Autodesk Inventor part; units mm, degrees
ref_plane "Arbeitsebene1" through (0, 0, 48) normal (0, 0, 1) x (1, 0, 0)
ref_plane "YZ Plane" through (0, 0, 0) normal (1, 0, 0) x (0, 1, 0)
ref_plane "XZ Plane" through (0, 0, 0) normal (0, 1, 0) x (-1, 0, 0)
sketch "Skizze1" plane through (0, 0, 0) normal (0, 0, 1) x (1, 0, 0)
  line L0 (0, 45) -> (110, 45)
  line L1 (110, 45) -> (110, 0)
  line L2 (110, 0) -> (0, 0)
  line L3 (0, 0) -> (0, 45)
  dimension "d0" = 110
  dimension "d1" = 45
extrude "Extrusion1" add sketch "Skizze1" along normal blind 12
sketch "Skizze2" plane through (110, 0, 0) normal (1, 0, 0) x (0, 0, -1)
  line L0 (0, 45) -> (-12, 45)
  line L1 (0, 45) -> (-62, 45)
  line L2 (-62, 45) -> (-62, 33)
  line L3 (-62, 33) -> (0, 33)
  line L4 (0, 33) -> (0, 45)
  point P0 (0, 0)
  dimension "d4" = 12
  dimension "d5" = 62
extrude "Extrusion2" add sketch "Skizze2" against normal up to surface (110 mm away)
fillet "Rundung1" radius 12 4 edges at (110, 0, 6) (0, 0, 6) (0, 39, 62) (110, 39, 62)
ref_plane "Arbeitsebene1" through (0, 0, 48) normal (0, 0, 1) x (1, 0, 0)
sketch "Skizze5" plane through (0, 0, 48) normal (0, 0, 1) x (1, 0, 0)
  line L0 (110, 45) -> (0, 45)
  line L1 (30, 45) -> (80, 45)
  line L2 (80, 45) -> (80, 10)
  line L3 (80, 10) -> (30, 10)
  line L4 (30, 10) -> (30, 45)
  line L5 (12, 0) -> (98, 0)
  point P0 (0, 0)
  point P1 (55, 10)
  point P2 (55, 0)
  dimension "d12" = 50
  dimension "d13" = 35
extrude "Extrusion4" add sketch "Skizze5" along normal up to surface (14 mm away)
sketch "Skizze3" plane through (0, 0, 12) normal (0, 0, 1) x (1, 0, 0)
  line L0 (98, 33) -> (12, 33)
  line L1 (44, 33) -> (66, 33)
  line L2 (66, 33) -> (66, 10)
  line L3 (66, 10) -> (44, 10)
  line L4 (44, 10) -> (44, 33)
  line L5 (12, 0) -> (98, 0)
  point P0 (0, 0)
  point P1 (55, 10)
  point P2 (55, 0)
  dimension "d9" = 22
  dimension "d10" = 23
sketch "Skizze9" plane through (0, 0, 48) normal (0, 0, -1) x (-1, 0, 0)
  line L0 (-80, 10) -> (-30, 10)
  line L1 (-35, 33) -> (-75, 33)
  line L2 (-75, 33) -> (-75, 10)
  line L3 (-75, 10) -> (-35, 10)
  line L4 (-35, 10) -> (-35, 33)
  line L5 (-98, 45) -> (-12, 45)
  point P0 (0, 0)
  point P1 (-55, 33)
  point P2 (-55, 45)
  dimension "d30" = 40
  dimension "d31" = 23
loft "Erhebung3" add profiles "Skizze3", "Skizze9"
sketch "Skizze10" plane through (30, 10, 62) normal (0, -1, 0) x (1, 0, 0)
  line L0 (68, 0) -> (-18, 0)
  arc A0 (10, 0) -> (40, 0) centre (25, 0) ccw
  line L1 (0, -14) -> (0, 0)
  line L2 (50, -14) -> (50, 0)
  point P0 (-30, -62)
  dimension "d38" = 30
  dimension "d39" = 10
extrude "Extrusion5" cut sketch "Skizze10" against normal up to surface (35 mm away)
sketch "Skizze11" plane through (0, 33, 12) normal (0, -1, 0) x (1, 0, 0)
  arc A0 (12, 50) -> (0, 38) centre (12, 38) ccw
  point P0 (0, -12)
hole "Bohrung1" at (12, 33, 50) direction (0, 1, 0) diameter 12 depth 12
sketch "Skizze12" plane through (110, 33, 12) normal (0, -1, 0) x (1, 0, 0)
  arc A0 (0, 38) -> (-12, 50) centre (-12, 38) ccw
  point P0 (-110, -12)
hole "Bohrung2" at (98, 33, 50) direction (0, 1, 0) diameter 12 depth 12
sketch "Skizze13" plane through (0, 0, 12) normal (0, 0, 1) x (1, 0, 0)
  arc A0 (98, 0) -> (110, 12) centre (98, 12) ccw
  point P0 (0, 0)
hole "Bohrung3" at (98, 12, 12) direction (0, 0, -1) diameter 12 depth 12
sketch "Skizze14" plane through (0, 0, 12) normal (0, 0, 1) x (1, 0, 0)
  arc A0 (0, 12) -> (12, 0) centre (12, 12) ccw
  point P0 (0, 0)
hole "Bohrung4" at (12, 12, 12) direction (0, 0, -1) diameter 12 depth 12
sketch "Skizze15" plane through (12, 0, 0) normal (0, -1, 0) x (1, 0, 0)
  line L0 (0, 0) -> (86, 0)
  line L1 (13, 0) -> (73, 0)
  line L2 (73, 0) -> (73, 8)
  line L3 (73, 8) -> (13, 8)
  line L4 (13, 8) -> (13, 0)
  line L5 (-12, 12) -> (-12, 0)
  dimension "d70" = 60
  dimension "d71" = 25
  dimension "d72" = 8
extrude "Extrusion6" cut sketch "Skizze15" against normal up to surface (45 mm away)
properties part number "manu" material "Stahl, galvanisiert"
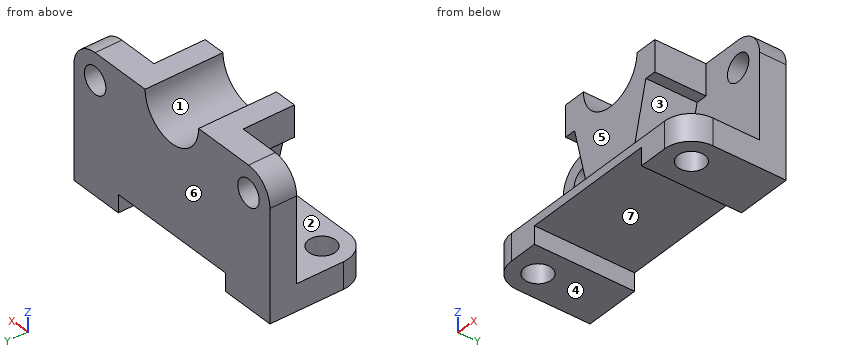
CAD build for the part. Positions are in the model's coordinates, mm. Face numbers are marked on the shaded views. A direction names the side the tool comes from. Coordinates: 2 decimals unless noted, no trailing zeros. Write each loop counter-clockwise with the first axis right and the second up, starting at its lowest first coordinate (ties: lowest second). Pieces come first, ordered by that corner, then holes. Notation, with made-up numbers: (-6, 83.5) -> (-1, 83.5) arc R23 cw to (-1, 122.5) -> close; hole circle Ø3 at (53, -10.75). An arc over 180 degrees is marked (long way). Return JSON: item names as keys, results as strings. Group by question number.
Q1. Cut at B-B, the plane y = 31. Give the cut face in (x, z).
Q2. Cut at C-C, the plane z = 31. Give the cut face in (x, y).
Q3. Pull direction Z, two halves, no side cores. Call the marked faces 1, 2, 3 and 4: released by +Z, released by -Z, zero draft, split by the parting line, or undercut.
Q4. Which spindle directions (+Z, -Z, +X, -X, +Y, -Y) get a long thin tool onto all of the face, cutting with end or side? Do the marked faces 5, 6 and 7. Say none if no direction does.
Q5. Drill centre lines: line 1 (X direction, y = 12, z = 9); line 2 (Y direction, x = 98, z = 6); line 3 (X direction, y = 42, z = 50). Where is each one in solid material? Low to high.
Q6. Cut at D-D, the plane x = 16. Give the cut face in (y, z), then the cut area to 3 significant figures.
Q7. Cut at A-A, the plane z = 6.5. Give the cut face in (x, y).
Q8. Flat gauge pins, fed straight in: pin 1 (1.5 mm diameter, centred on x = 33.5, y = 23.5, fed in from -Z); pin 2 (7 mm diameter, centred on x = 12, y = 12, fed in from +Z); pin 3 (19 mm diameter, centred on x = 98, y = 12, fed in from +Z); pin 4 (10 mm diameter, centred on x = 72, z = 53, fed in from -Y). Where does each tip first touch, or does it go through?
Returned:
{
 "1": {"outline": "(0, 0) -> (25, 0) -> (25, 8) -> (85, 8) -> (85, 0) -> (110, 0) -> (110, 12) -> (66, 12) -> (75, 48) -> (80, 48) -> (80, 62) -> (70, 62) arc R15 cw to (40, 62) -> (30, 62) -> (30, 48) -> (35, 48) -> (44, 12) -> (0, 12) -> close"},
 "2": {"outline": "(0, 33) -> (39.25, 33) -> (39.25, 10) -> (70.75, 10) -> (70.75, 33) -> (110, 33) -> (110, 45) -> (0, 45) -> close"},
 "3": {"face 1": "released by +Z", "face 2": "undercut", "face 3": "undercut", "face 4": "released by -Z"},
 "4": {"face 5": "+Z, +X, -X, -Y", "face 6": "+Z, -Z, +X, -X, +Y", "face 7": "-Z, +Y, -Y"},
 "5": {"line 1": "x = 0 to 6, 18 to 92, 104 to 110", "line 2": "y = 0 to 6, 18 to 45", "line 3": "x = 0 to 6, 18 to 46, 64 to 92, 104 to 110"},
 "6": {"outline": "(0, 0) -> (7.53, 0) -> (7.53, 12) -> (0, 12) -> close; (16.47, 0) -> (45, 0) -> (45, 45.53) -> (33, 45.53) -> (33, 12) -> (16.47, 12) -> close; (33, 54.47) -> (45, 54.47) -> (45, 62) -> (33, 62) -> close", "area": "925 mm2"},
 "7": {"outline": "(0, 12) arc R12 ccw to (12, 0) -> (25, 0) -> (25, 45) -> (0, 45) -> close; (85, 0) -> (98, 0) arc R12 ccw to (110, 12) -> (110, 45) -> (85, 45) -> close; hole circle Ø12 at (12, 12); hole circle Ø12 at (98, 12)"},
 "8": {"pin 1": "stops at z = 8", "pin 2": "passes through", "pin 3": "stops at z = 12", "pin 4": "stops at y = 10"}
}
